Input: part model. Units: mm. Frame: model coordinates. Give positions to 0.01 mm unless a question says otherwise; leave off trailing zeros. Order: outer loops, then holes, each group sorted by start corner. A loop starts at its lowest first (then second) coordinate and runs counter-clockwise, first axis right, second up. Notation, with made-up numbers: (-18, -21.5) -> (19, -21.5) arc R14 ccw to (19, -4.5) -> close; hole circle Ø10 at (-33.75, -25). An arc over 180 degrees is marked (long way). Use a Markdown table: item, result. Add a question column.
from build123d import *

# Parameters (mm, degrees)
SKETCH_R  = 1.6
PAD_DEPTH = 5


with BuildPart() as part:
    # Sketch → Pad (new body)
    with BuildSketch(Plane.XY):
        with BuildLine():
            ThreePointArc((-38.25, 7.75), (-43.25, 12.75), (-48.25, 7.75))
            Line((-48.25, 7.75), (-48.25, -71))
            Line((-48.25, -71), (54.088146, -71))
            Line((54.088146, -61), (54.088146, -71))
            Line((48.25, -61), (54.088146, -61))
            Line((48.25, 7.75), (48.25, -61))
            ThreePointArc((48.25, 7.75), (43.25, 12.75), (38.25, 7.75))
            Line((38.25, 7.75), (38.25, -61))
            Line((-38.25, -61), (38.25, -61))
            Line((-38.25, 7.75), (-38.25, -61))
        make_face()
        with Locations((-43.25, 7.75)):
            Circle(SKETCH_R, mode=Mode.SUBTRACT)
        with Locations((43.25, 7.75)):
            Circle(SKETCH_R, mode=Mode.SUBTRACT)
        with Locations((-43.25, -25.25)):
            Circle(SKETCH_R, mode=Mode.SUBTRACT)
        with Locations((43.25, -25.25)):
            Circle(SKETCH_R, mode=Mode.SUBTRACT)
        with Locations((7.5, -66)):
            Circle(SKETCH_R, mode=Mode.SUBTRACT)
        with Locations((-9, -66)):
            Circle(SKETCH_R, mode=Mode.SUBTRACT)
        with Locations((30.5, -66)):
            Circle(SKETCH_R, mode=Mode.SUBTRACT)
        with Locations((47, -66)):
            Circle(SKETCH_R, mode=Mode.SUBTRACT)
    extrude(amount=PAD_DEPTH)


solid = part.part
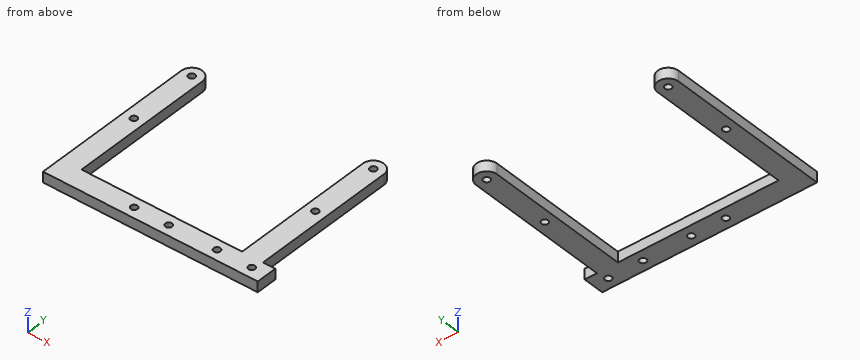
Q1. Section query D-D (x = 15). Return loops of the section in (y, z).
Q2. Ray query, line 1 (Y direction, x = -43.25, z = 3.1); line 2 (X direction, y = -66, z = 3.05); line 3 (X direction, y = -9, z = 0.9). Return the intervals inside material, ascending.
Q3. Section query B-B (z = 3.45). Give the number of separate pieces and of enclosed holes in the cut face, plus the area to 3 significant figures.
Q4. Section query C-C (x = 30.5). Return loops of the section in (y, z), plus the area to 3 significant figures.
Q5. First-contact query: pin 1 (2.5 mm diameter, centred on x = 52, z = 3, fed in from +Y). Flat tip, straight axial feed; report the tip coordinate or a pass-through.
Q6. Section query A-A (y = -45). Return loops of the section in (x, z), plus the area to 3 significant figures.
Solution:
| question | item | result |
|---|---|---|
| 1 | outline | (-71, 0) -> (-61, 0) -> (-61, 5) -> (-71, 5) -> close |
| 2 | line 1 | y = -71 to -26.85, -23.65 to 6.15, 9.35 to 12.75 |
| 2 | line 2 | x = -48.25 to -10.6, -7.4 to 5.9, 9.1 to 28.9, 32.1 to 45.4, 48.6 to 54.09 |
| 2 | line 3 | x = -48.25 to -38.25, 38.25 to 48.25 |
| 3 | separate pieces | 1 |
| 3 | enclosed holes | 8 |
| 3 | area | 2,410 mm² |
| 4 | outline | (-71, 0) -> (-67.6, 0) -> (-67.6, 5) -> (-71, 5) -> close; (-64.4, 0) -> (-61, 0) -> (-61, 5) -> (-64.4, 5) -> close |
| 4 | area | 34.0 mm² |
| 5 | pin 1 | stops at y = -61 |
| 6 | outline | (-48.25, 0) -> (-38.25, 0) -> (-38.25, 5) -> (-48.25, 5) -> close; (38.25, 0) -> (48.25, 0) -> (48.25, 5) -> (38.25, 5) -> close |
| 6 | area | 100 mm² |
